CAD build for the part. Positions are in the model's coordinates, mm. Round coordinates to 2 decimals unless told otherwise and drop trailing zeros. Write each loop counter-clockwise with the first axis right and the second up, starting at its lowest first coordinate (ties: lowest second). Pieces come first, ordered by that corner, then holes. Notation, with made-up numbers: M 41.5,38.5 L 95.5,38.5 A16 ccw 95.5,65.5 Z; hole C 27,-25.5 d1. An arc over 180 degrees is marked long. Write each question's results on one line, items separated by ' | '. Start each with the question number.
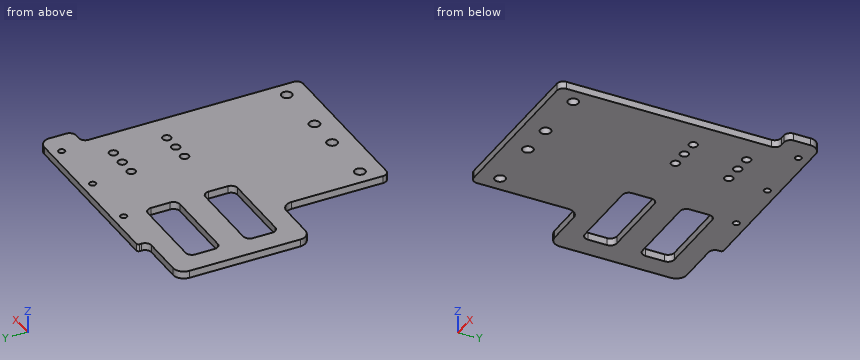
```python
from build123d import *

# Parameters (mm, degrees)
MODEL_R         = 2.5
MODEL_R_2       = 2
MODEL_R_3       = 1.5
EXTRUDE_1_DEPTH = 3.45


with BuildPart() as part:
    # Model → 凸台-拉伸1 (new body)
    with BuildSketch(Plane.XY):
        with BuildLine():
            Line((123.577210347, 109.56127227), (123.577210347, 117.42565066))
            ThreePointArc((123.577210347, 117.42565066), (122.112744253, 120.961184566), (118.577210347, 122.42565066))
            Line((118.577210347, 122.42565066), (35.577210347, 122.42565066))
            ThreePointArc((35.577210347, 122.42565066), (34.870103566, 122.132757441), (34.577210347, 121.42565066))
            Line((34.577210347, 121.42565066), (34.577210347, 120.42565066))
            ThreePointArc((34.577210347, 120.42565066), (33.69853069, 118.304330316), (31.577210347, 117.42565066))
            Line((31.577210347, 117.42565066), (11.977210347, 117.42565066))
            ThreePointArc((11.977210347, 117.42565066), (8.441676441, 115.961184566), (6.977210347, 112.42565066))
            Line((6.977210347, 112.42565066), (6.977210347, 60.42565066))
            ThreePointArc((6.977210347, 60.42565066), (8.441676441, 56.890116754), (11.977210347, 55.42565066))
            Line((11.977210347, 55.42565066), (29.077210347, 55.42565066))
            ThreePointArc((29.077210347, 55.42565066), (32.612744253, 53.961184566), (34.077210347, 50.42565066))
            Line((34.077210347, 50.42565066), (34.077210347, 7.54555066))
            ThreePointArc((34.077210347, 7.54555066), (34.955890003, 5.424230316), (37.077210347, 4.54555066))
            Line((37.077210347, 4.54555066), (112.077210347, 4.54555066))
            ThreePointArc((112.077210347, 4.54555066), (114.19853069, 5.424230316), (115.077210347, 7.54555066))
            Line((115.077210347, 7.54555066), (115.077210347, 103.56127227))
            ThreePointArc((115.077210347, 103.56127227), (115.955890003, 105.682592613), (118.077210347, 106.56127227))
            Line((118.077210347, 106.56127227), (120.577210347, 106.56127227))
            ThreePointArc((120.577210347, 106.56127227), (122.69853069, 107.439951926), (123.577210347, 109.56127227))
        make_face()
        with Locations((82.577210347, 14.54555066)):
            Circle(MODEL_R, mode=Mode.SUBTRACT)
        with Locations((107.577210347, 14.54555066)):
            Circle(MODEL_R, mode=Mode.SUBTRACT)
        with Locations((101.477210347, 98.92565066)):
            Circle(MODEL_R_2, mode=Mode.SUBTRACT)
        with Locations((93.477210347, 98.92565066)):
            Circle(MODEL_R_2, mode=Mode.SUBTRACT)
        with Locations((85.477210347, 98.92565066)):
            Circle(MODEL_R_2, mode=Mode.SUBTRACT)
        with Locations((93.477210347, 73.92565066)):
            Circle(MODEL_R_2, mode=Mode.SUBTRACT)
        with Locations((101.477210347, 73.92565066)):
            Circle(MODEL_R_2, mode=Mode.SUBTRACT)
        with Locations((85.477210347, 73.92565066)):
            Circle(MODEL_R_2, mode=Mode.SUBTRACT)
        with Locations((84.577210347, 117.42565066)):
            Circle(MODEL_R_3, mode=Mode.SUBTRACT)
        with Locations((112.577210347, 117.42565066)):
            Circle(MODEL_R_3, mode=Mode.SUBTRACT)
        with Locations((56.577210347, 117.42565066)):
            Circle(MODEL_R_3, mode=Mode.SUBTRACT)
        with Locations((41.577210347, 14.54555066)):
            Circle(MODEL_R, mode=Mode.SUBTRACT)
        with Locations((66.577210347, 14.54555066)):
            Circle(MODEL_R, mode=Mode.SUBTRACT)
        with BuildLine():
            Line((53.977210347, 65.42565066), (19.977210347, 65.42565066))
            ThreePointArc((19.977210347, 65.42565066), (17.855890003, 66.304330316), (16.977210347, 68.42565066))
            Line((16.977210347, 68.42565066), (16.977210347, 77.42565066))
            ThreePointArc((16.977210347, 77.42565066), (17.855890003, 79.546971003), (19.977210347, 80.42565066))
            Line((19.977210347, 80.42565066), (53.977210347, 80.42565066))
            ThreePointArc((53.977210347, 80.42565066), (56.09853069, 79.546971003), (56.977210347, 77.42565066))
            Line((56.977210347, 77.42565066), (56.977210347, 68.42565066))
            ThreePointArc((56.977210347, 68.42565066), (56.09853069, 66.304330316), (53.977210347, 65.42565066))
        make_face(mode=Mode.SUBTRACT)
        with BuildLine():
            Line((53.977210347, 107.42565066), (19.977210347, 107.42565066))
            ThreePointArc((19.977210347, 107.42565066), (17.855890003, 106.546971003), (16.977210347, 104.42565066))
            Line((16.977210347, 104.42565066), (16.977210347, 95.42565066))
            ThreePointArc((16.977210347, 95.42565066), (17.855890003, 93.304330316), (19.977210347, 92.42565066))
            Line((19.977210347, 92.42565066), (53.977210347, 92.42565066))
            ThreePointArc((53.977210347, 92.42565066), (56.09853069, 93.304330316), (56.977210347, 95.42565066))
            Line((56.977210347, 95.42565066), (56.977210347, 104.42565066))
            ThreePointArc((56.977210347, 104.42565066), (56.09853069, 106.546971003), (53.977210347, 107.42565066))
        make_face(mode=Mode.SUBTRACT)
    extrude(amount=EXTRUDE_1_DEPTH)


solid = part.part
```
1) Wall check: line 1 along Y through (x, z) = (37, 1.65); line 2 along Y through (x, z) = (112.5, 1.8); line 3 along X through (y, z) = (77.5, 1.2). Give the ranges that are in metal, low to high. Write a range as from..to.
2) Drop flat-ended pins along their axis: pin 1 Ø12 at (x, y) = (100.5, 72) entering from -Z; pin 2 Ø1 at (y, z) = (50.5, 1.5) entering from +X; pin 3 Ø6 at (x, y) = (44, 69) entering from -Z; pin 4 Ø1.1 at (y, z) = (121, 1.5) entering from -X. Give the stop position or say it passes through.
3) Saw through at B-B, the plane x = 116.5. Write the cut outline in (y, z), plus the area to 3 significant figures.
4) Saw through at C-C, the plane z = 2.75. State how many separate pieces and enclosed holes the cut face has, plus the area to 3 significant figures.
5) Saw through at A-A, the plane y = 86. Write the cut outline in (x, z).
Filled sheet:
1) line 1: y = 4.55..65.43, 80.43..92.43, 107.43..122.43 | line 2: y = 4.58..115.93, 118.92..122.43 | line 3: x = 6.98..16.98, 56.98..115.08
2) pin 1: stops at z = 0 | pin 2: stops at x = 115.08 | pin 3: passes through | pin 4: stops at x = 34.58
3) outline: M 106.11,0 L 122.43,0 L 122.43,3.45 L 106.11,3.45 Z | area: 56.3 mm^2
4) separate pieces: 1 | enclosed holes: 15 | area: 9,990 mm^2
5) outline: M 6.98,0 L 115.08,0 L 115.08,3.45 L 6.98,3.45 Z
